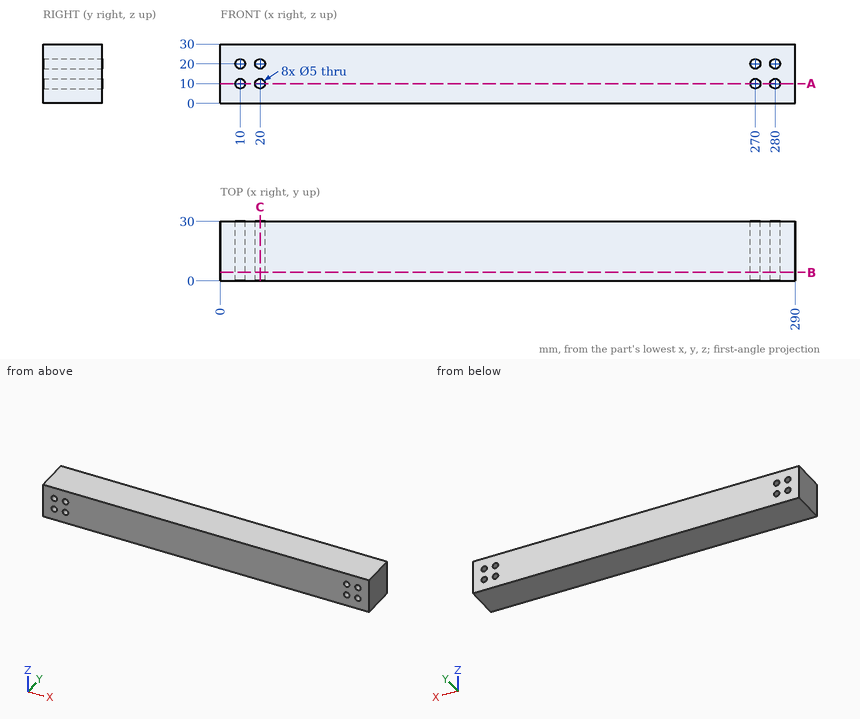
Part print with two shaded views. Sizes in mm from the minimum x, y, z corner. Round coordinates to 2 decimals unless told otherwise and drop trailing zeros. Write each loop counter-clockwise with the first axis right and the second up, starting at its lowest first coordinate (ties: lowest second). Pieces come first, ordered by that corner, then holes. Notation, with made-up numbers: (6.5, 57) -> (51.5, 57) arc R21 ccw to (51.5, 79) -> close; hole circle Ø2 at (58.5, -19). An arc over 180 degrees is marked (long way). Put each result on its own line as item: value.
Item 1: Flat gauge pin, fed straight in: P1, Ø3, axis at y = 21, z = 22, coming from the -X side. Where does the tip first touch, or does it go through?
Here are the results:
P1: stops at x = 0
Item 2: Wall check: probe 1 along Z at (x, y) = (20, 9); probe 2 along X at (y, z) = (23.5, 19); probe 3 along Z at (x, y) = (272, 25.5). Give the ranges that are in metal, low to high. Write a range as from..to.
Here are the results:
probe 1: z = 0..7.5, 12.5..17.5, 22.5..30
probe 2: x = 0..7.71, 12.29..17.71, 22.29..267.71, 272.29..277.71, 282.29..290
probe 3: z = 0..8.5, 11.5..18.5, 21.5..30
Item 3: Slice it at A-A, the plane z = 10. Give the cut face in (x, y).
Here are the results:
outline: (0, 0) -> (7.5, 0) -> (7.5, 30) -> (0, 30) -> close; (12.5, 0) -> (17.5, 0) -> (17.5, 30) -> (12.5, 30) -> close; (22.5, 0) -> (267.5, 0) -> (267.5, 30) -> (22.5, 30) -> close; (272.5, 0) -> (277.5, 0) -> (277.5, 30) -> (272.5, 30) -> close; (282.5, 0) -> (290, 0) -> (290, 30) -> (282.5, 30) -> close
Item 4: Slice it at B-B, the plane y = 4.25. Count the separate pieces of the cut face and the enclosed holes in it, plus the area to 3 significant figures.
Here are the results:
separate pieces: 1
enclosed holes: 8
area: 8,540 mm^2
Item 5: Slice it at C-C, the plane x = 20. Give the cut face in (y, z), plus the area to 3 significant figures.
Here are the results:
outline: (0, 0) -> (30, 0) -> (30, 7.5) -> (0, 7.5) -> close; (0, 12.5) -> (30, 12.5) -> (30, 17.5) -> (0, 17.5) -> close; (0, 22.5) -> (30, 22.5) -> (30, 30) -> (0, 30) -> close
area: 600 mm^2
